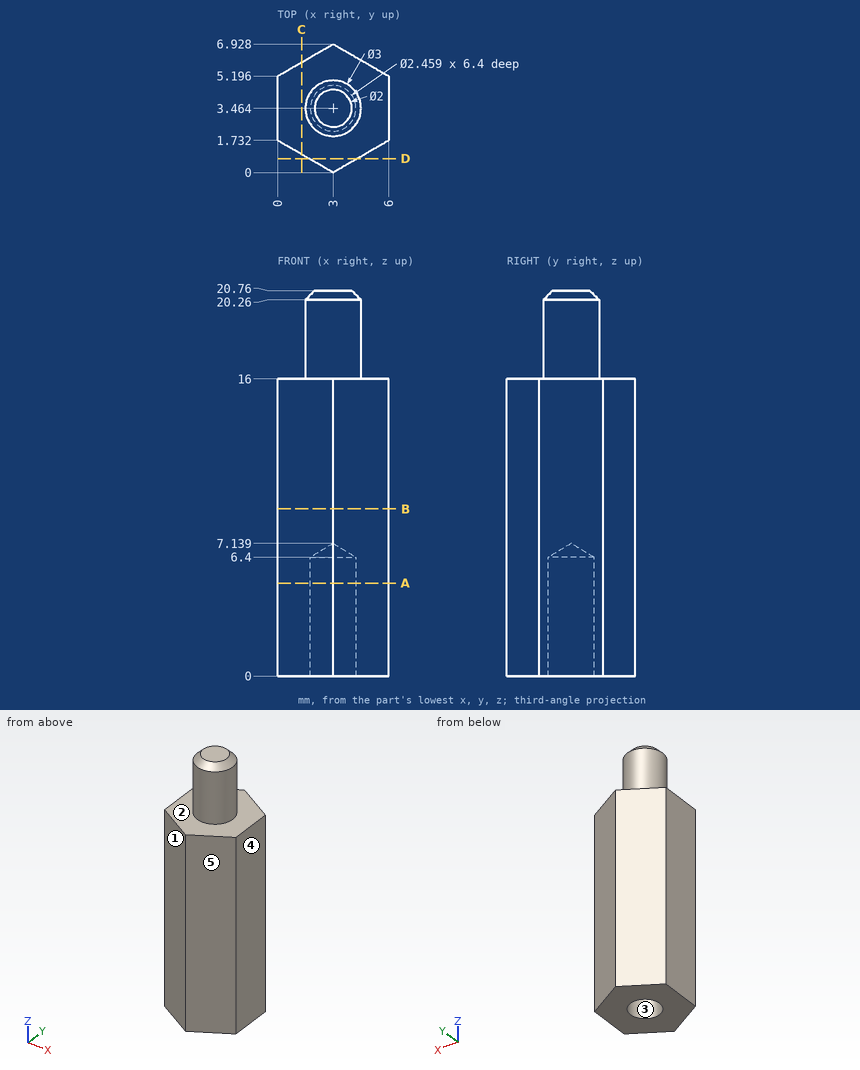
Verification items for this drawing (mm, ordinates from the low corner). A direction names the side the tool comes from. Round coordinates to 2 decimals unless told otherwise and drop trailing zeros. Order: outer loops, then holes, each group sorted by start corner. A loop starts at its lowest first (then second) coordinate and runs counter-clockwise, first axis right, second up. Notation, with made-up numbers: (19.25, 78) -> (73.25, 78) arc R7 ccw to (73.25, 89) -> close; hole circle Ø9 at (55, 32.5). An arc over 180 degrees is marked (long way). Use one line per item in the form item = value.
1. Cross-section at C-C, the plane x = 1.3. Enter the section's corners in (y, z).
Working result:
outline = (0.98, 0) -> (5.95, 0) -> (5.95, 16) -> (0.98, 16) -> close
2. Cross-section at A-A, the plane z = 5. Enter the section's corners in (x, y).
Working result:
outline = (0, 1.73) -> (3, 0) -> (6, 1.73) -> (6, 5.2) -> (3, 6.93) -> (0, 5.2) -> close; hole circle Ø2.46 at (3, 3.46)
3. Cross-section at B-B, the plane z = 9. Enter the section's corners in (x, y), plus the area to 3 significant figures.
Working result:
outline = (0, 1.73) -> (3, 0) -> (6, 1.73) -> (6, 5.2) -> (3, 6.93) -> (0, 5.2) -> close
area = 31.2 mm^2
4. Set-up check for the marked faces 1 and 2: record each of +Z, -Z, +X, -X, +Y, -Y from which the full face is reachable in a straight line by a thin tool's end or side.
Working result:
face_1 = +Z, -Z, -X, -Y
face_2 = +Z
5. Scan lines: line 1 along Z through (x, y) = (1.3, 2); line 2 along X through (y, z) = (4.5, 2.5); line 3 along X through (y, z) = (3, 2.5). Record each from-to range of solid material in increasing order. Write a range as from..to.
Working result:
line_1 = 0..16
line_2 = 0..2.34, 3.66..6
line_3 = 0..1.86, 4.14..6
6. Mould release check, pull along Y, two halves, no side actions. Record for the marked faces 3, 4 and 5: pulls with the +Y half, pulls with the -Y half, needs draft (parallel to the pull), parting line crosses it, or undercut.
Working result:
face_3 = undercut
face_4 = needs draft
face_5 = pulls with the -Y half
7. Cross-section at D-D, the plane y = 0.75. Enter the section's corners in (x, z).
Working result:
outline = (1.7, 0) -> (4.3, 0) -> (4.3, 16) -> (1.7, 16) -> close
